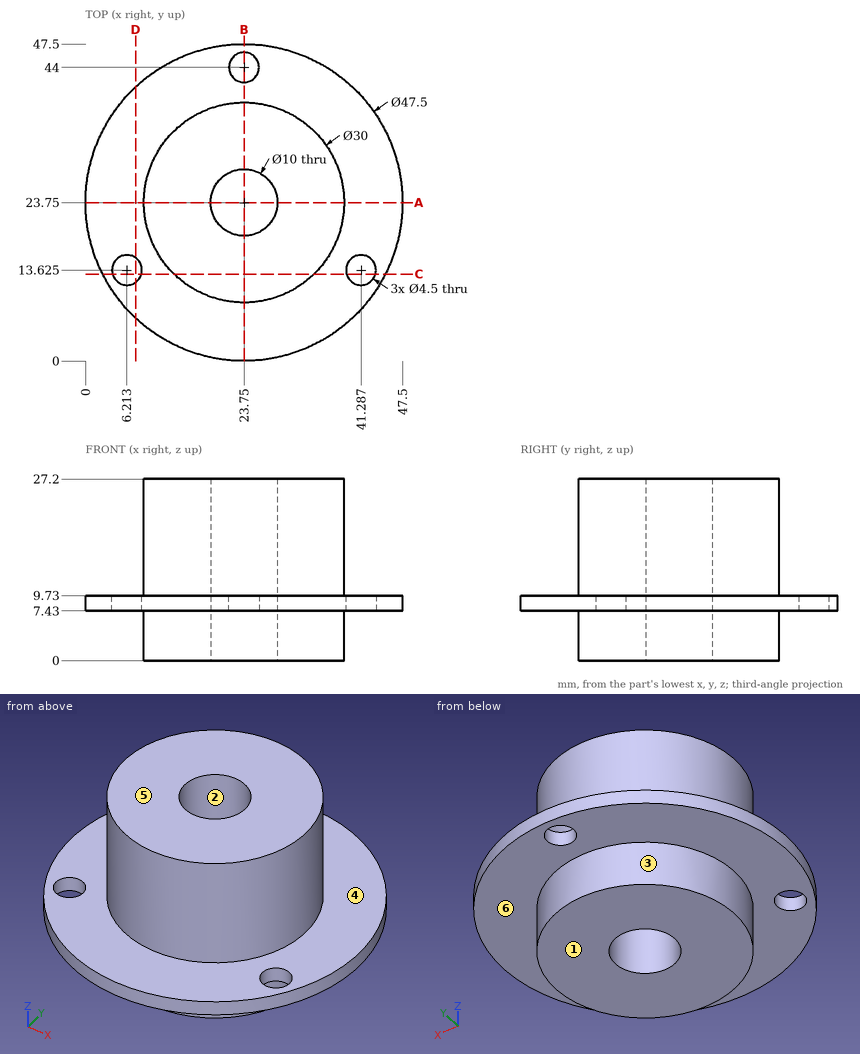
Design review of the part shown in the three views and the two pictorial views. Dimensions are in mm from the part's minimum x, y and z. A direction names the side the tool comes from. Give positions to 0.01 mm unless a question says otherwise; leave off trailing zeros. Write each loop counter-clockwise with the first axis right and the second up, starting at its lowest first coordinate (ties: lowest second). Pieces come first, ordered by that corner, then holes. Notation, with made-up numbers: (20, -23.5) - (69, -23.5) arc R29 ccw to (69, 8.5) - close; hole circle Ø6 at (-37.75, -17.75). An arc over 180 degrees is marked (long way). Return JSON: item names as keys, results as strings. Group by question number.
(1) We need section D-D, the plane x = 7.5. Give the boundary of the cut face in (y, z), then the cut area to 3 significant figures.
(2) We need section C-C, the plane y = 13. Give the boundary of the cut face in (x, z), then the cut area to 4 significant figures.
(3) Mouldability with a two-part tool opening along Y and no side actions: class the marked faces 1, 2 and 3 as +Y half, -Y half, draft (parallel to the pull), parting line (faces both ways), or undercut.
(4) We need section B-B, the plane x = 23.75. Give the boundary of the cut face in (y, z).
(5) Machinability: for the marked faces 4, 5 and 6, which of the approach directions +Z, -Z, +X, -X, +Y, -Y give a long, thin tool a straight path to every point of the face, cutting with its end or side? Answer none if there is none.
(6) To check wall thickness, follow probe 1 along Y at (x, z) = (23.75, 8.55); probe 2 along Z at (x, y) = (39.5, 18); probe 3 along Y at (x, z) = (23.75, 10.75). State the ranges of each line that lie inside material, in increasing order.
(7) Insertion check: pin 1 (8 mm diameter, centred on x = 19, z = 23, fed in from -Y); pin 2 (12 mm diameter, centred on x = 11, z = 6.5, fed in from +Y); pin 3 (2.5 mm diameter, centred on x = 23.75, y = 44, fed in from +Z); pin 4 (6 mm diameter, centred on x = 13.5, z = 20.5, fed in from -Y). Each pin has a flat end and moves straight along its axis. Give the tip position at first contact, or say it passes through.
(8) We need section A-A, the plane y = 23.75. Give the boundary of the cut face in (x, z).
Reported:
{
 "1": {"outline": "(6.43, 7.43) - (11.78, 7.43) - (11.78, 9.73) - (6.43, 9.73) - close; (15.47, 7.43) - (41.07, 7.43) - (41.07, 9.73) - (15.47, 9.73) - close", "area": "71.2 mm2"},
 "2": {"outline": "(2.57, 7.43) - (4.05, 7.43) - (4.05, 9.73) - (2.57, 9.73) - close; (8.37, 7.43) - (13.29, 7.43) - (13.29, 0) - (34.21, 0) - (34.21, 7.43) - (39.13, 7.43) - (39.13, 9.73) - (34.21, 9.73) - (34.21, 27.2) - (13.29, 27.2) - (13.29, 9.73) - (8.37, 9.73) - close; (43.45, 7.43) - (44.93, 7.43) - (44.93, 9.73) - (43.45, 9.73) - close", "area": "598.5 mm2"},
 "3": {"face 1": "draft", "face 2": "undercut", "face 3": "parting line"},
 "4": {"outline": "(0, 7.43) - (8.75, 7.43) - (8.75, 0) - (18.75, 0) - (18.75, 27.2) - (8.75, 27.2) - (8.75, 9.73) - (0, 9.73) - close; (28.75, 0) - (38.75, 0) - (38.75, 7.43) - (41.75, 7.43) - (41.75, 9.73) - (38.75, 9.73) - (38.75, 27.2) - (28.75, 27.2) - close; (46.25, 7.43) - (47.5, 7.43) - (47.5, 9.73) - (46.25, 9.73) - close"},
 "5": {"face 4": "+Z", "face 5": "+Z, +X, -X, +Y, -Y", "face 6": "-Z"},
 "6": {"probe 1": "y = 0 to 18.75, 28.75 to 41.75, 46.25 to 47.5", "probe 2": "z = 7.43 to 9.73", "probe 3": "y = 8.75 to 18.75, 28.75 to 38.75"},
 "7": {"pin 1": "stops at y = 8.77", "pin 2": "stops at y = 46.5", "pin 3": "passes through", "pin 4": "stops at y = 10.62"},
 "8": {"outline": "(0, 7.43) - (8.75, 7.43) - (8.75, 0) - (18.75, 0) - (18.75, 27.2) - (8.75, 27.2) - (8.75, 9.73) - (0, 9.73) - close; (28.75, 0) - (38.75, 0) - (38.75, 7.43) - (47.5, 7.43) - (47.5, 9.73) - (38.75, 9.73) - (38.75, 27.2) - (28.75, 27.2) - close"}
}
